Design review of the part built by this model. Coordinates are the model's own, in mm. Give positions to 0.01 mm unless a question says otherwise; leave off trailing zeros. Order: outer loops, then holes, each group sorted by start corner. A loop starts at its lowest first (then second) coordinate and runs counter-clockwise, first axis right, second up.
```python
from build123d import *

# Parameters (mm, degrees)
F0_W     = 500
F0_H     = 40
F1_DEPTH = 5
F3_DEPTH = 500
F5_DEPTH = 500


with BuildPart() as f1:
    # F0 (on Top) → F1 (new body)
    with BuildSketch(Plane.XY):
        Rectangle(F0_W, F0_H)
    extrude(amount=F1_DEPTH)

    # F2 (on face) → F3 (join, through all)
    with BuildSketch(Plane.YZ.offset(250)):
        Polygon((-9.25, 11.7), (-9.25, 0), (9.25, 0), (9.25, 11.7), (6.4414839943, 11.7), (-6.4414839943, 11.7), align=None)
        with BuildLine():
            Line((-6.3045076751, 11.9828207053), (-6.4414839943, 11.7))
            Line((-6.4414839943, 11.7), (6.4414839943, 11.7))
            Line((6.4414839943, 11.7), (5.346455176, 13.9609515597))
            Line((5.346455176, 13.9609515597), (3.4871191548, 17.8))
            ThreePointArc((3.4871191548, 17.8), (0, 17), (-3.4871191548, 17.8))
            Line((-3.4871191548, 17.8), (-6.3045076751, 11.9828207053))
        make_face()
    extrude(amount=-F3_DEPTH)

    # F4 (on face) → F5 (join, through all)
    with BuildSketch(Plane(origin=(-250, 0, 0), x_dir=(0, -1, 0), z_dir=(-1, 0, 0))):
        with BuildLine():
            ThreePointArc((3.4871191548, 17.8), (6.7785305649, 20.7512915632), (8, 25))
            ThreePointArc((8, 25), (-4.2487084368, 31.7785305649), (-3.4871191548, 17.8))
            ThreePointArc((-3.4871191548, 17.8), (0, 17), (3.4871191548, 17.8))
        make_face()
    extrude(amount=-F5_DEPTH)


solid = f1.part
```
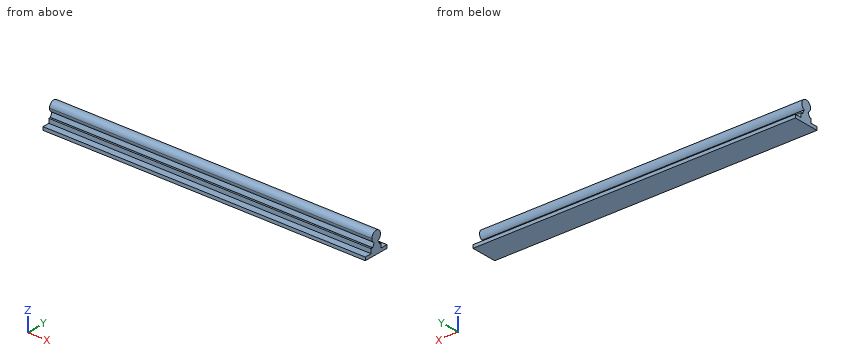
1. For pin 1 (3 mm diameter, centred on x = 82.5, y = -8, fed in from +Z); pin 2 (2 mm diameter, centred on x = -162, z = 16.5, fed in from -Y); pin 3 (3 mm diameter, centred on x = -53, y = 7.5, fed in from +Z), all flat-tipped, find the tip position at first contact; note any pin that passes through.
Recorded:
pin 1: stops at z = 29.66
pin 2: stops at y = -4.6
pin 3: stops at z = 30.29
2. Take a section at A-A (x = -186.5). State the section outline as (y, z) points.
Recorded:
outline: (-20, 0) - (20, 0) - (20, 5) - (9.25, 5) - (9.25, 11.7) - (6.44, 11.7) - (3.49, 17.8) arc R8 ccw (long way) to (-3.49, 17.8) - (-6.44, 11.7) - (-9.25, 11.7) - (-9.25, 5) - (-20, 5) - close
3. For line 1 along Z through (x, y) = (-66, 9.5); line 2 along Z through (x, y) = (72.5, -1); line 3 along Z through (x, y) = (-202, -4), list the stretches that pass through material, from the lowest coordinate up.
Recorded:
line 1: z = 0 to 5
line 2: z = 0 to 32.94
line 3: z = 0 to 16.74, 18.07 to 31.93
4. Take a section at B-B (y = 14.5). State the section outline as (x, z) points, then the cut area to 3 significant figures.
Recorded:
outline: (-250, 0) - (250, 0) - (250, 5) - (-250, 5) - close
area: 2,500 mm2
